Verification items for the finished model (mm, model axes). A direction names the side the tool comes from. Coordinates: 2 decimals unless noted, no trailing zeros. Write each loop counter-clockwise with the first axis right and the second up, starting at its lowest first coordinate (ties: lowest second). Pieces come first, ordered by that corner, then holes.
```python
from build123d import *

# Parameters (mm, degrees)
BASPROSKE_W          = 6
BASPROSKE_H          = 22
TOOTHCUT_DEPTH       = 32.685959036
TEETHCUTS_COUNT      = 20
TEETHCUTS_ANGLE      = 342
HUBNEAONESKE_R       = 11
HUBNEARONE_DEPTH     = 6.2500508
BORSKE_R             = 4
BORE_DEPTH           = 12.2500508
M2_CLEARANCE_HOLE1_D = 2.2


with BuildPart() as part:
    # BasProSke → Base-Revolve (revolve)
    with BuildSketch(Plane(origin=(0, 0, 0), x_dir=(1, 0, 0), z_dir=(0, 1, 0)), mode=Mode.PRIVATE) as base_revolve_sk:
        with Locations((3, 11)):
            Rectangle(BASPROSKE_W, BASPROSKE_H)
    revolve(base_revolve_sk.sketch.rotate(Axis((-10, 0, 0), (1, 0, 0)), 180), axis=Axis((-10, 0, 0), (1, 0, 0)))

    # TooCutSke → ToothCut (cut, through all)
    with BuildSketch(Plane(origin=(0, 0, 0), x_dir=(0, 0, -1), z_dir=(1, 0, 0))):
        with BuildLine():
            ThreePointArc((0.986171591, 17.471189616), (0, 17.499), (-0.986171591, 17.471189616))
            ThreePointArc((-0.986171591, 17.471189616), (-1.626916196, 19.798789858), (-2.932850173, 21.829260982))
            ThreePointArc((-2.932850173, 21.829260982), (0, 22.0254), (2.932850173, 21.829260982))
            ThreePointArc((2.932850173, 21.829260982), (1.626916196, 19.798789858), (0.986171591, 17.471189616))
        make_face()
    toothcut = extrude(amount=TOOTHCUT_DEPTH, mode=Mode.SUBTRACT)

    # TeethCuts: ToothCut ×20 about axis
    teethcuts_axis = Axis((-10, 0, 0), (1, 0, 0))
    for i in range(1, TEETHCUTS_COUNT):
        add(toothcut.rotate(teethcuts_axis, i * TEETHCUTS_ANGLE / (TEETHCUTS_COUNT - 1)), mode=Mode.SUBTRACT)

    # HubNeaOneSke → HubNearOne (add)
    with BuildSketch(Plane.ZY):
        with Locations(Location((0, 0, 0), (0, 0, 180))):
            Circle(HUBNEAONESKE_R)
    extrude(amount=HUBNEARONE_DEPTH)

    # BorSke → Bore (cut, symmetric)
    with BuildSketch(Plane(origin=(0, 0, 0), x_dir=(0, 0, -1), z_dir=(1, 0, 0))):
        with Locations(Location((0, 0, 0), (0, 0, 180))):
            Circle(BORSKE_R)
    extrude(amount=BORE_DEPTH, both=True, mode=Mode.SUBTRACT)

    # M2 Clearance Hole1 (through all)
    with Locations(Plane(origin=(6, 0, 0), x_dir=(0, 0, -1), z_dir=(1, 0, 0))):
        with Locations((0, 8), (5.656854249, 5.656854249), (8, 0), (5.656854249, -5.656854249), (0, -8), (-5.656854249, -5.656854249), (-8, 0), (-5.656854249, 5.656854249)):
            Hole(M2_CLEARANCE_HOLE1_D / 2)


solid = part.part
```
1. Sectioned sample at C-C, the plane z = -8. Record the boundary of the cut face in (x, y).
2. Material ranges on L1, parallel to Y at x = -2.75, z = 0; L2, parallel to Z at x = -1.25, y = 5; L3, parallel to Y at x = -5, z = 1, recorded low to high.
3. Gauge pin test, flat ends, axial feed: P1, Ø6, axis at y = -5.5, z = 17, coming from the -X side; P2, Ø5, axis at x = 0, y = 10, coming from the +Z side; P3, Ø4, axis at x = -4, y = 7, coming from the -Z side. Record the tip position at first contact, or that the pin passes through.
4. Sectioned sample at D-D, the plane x = -2.75. Give the number of separate pieces and of enclosed holes in the cut face, and give its area (3 significant figures).
5. Sectioned sample at A-A, the plane y = 0. Record the boundary of the cut face in (x, z).
6. Draft check along Y on faces 1 (the flat face through (6, 5, 0)), 2 (the cylindrical face through (-0.211, 6.747, -5.8)), 3 (the cylindrical face through (2.96, 7.63, -18.29)), 4 (the cylindrical face through (3.04, -9.99, -19.6)). Enter one of: pulls with the +Y half, pulls with the -Y half, needs draft (parallel to the pull), parting line crosses it, or undercut.
7. Tool access check on faces 5 (the cylindrical face through (2.96, -4.57, 19.35)), 6 (the cylindrical face through (2.96, 18.29, 7.63)), 7 (the cylindrical face through (2.958, -7.678, -18.341)). Record the directions out of +Z, -Z, +X, -X, +Y, -Y that give a thin tool (end or side, any length) a straight path to the whole face; none if there is none.
Outcome:
1. outline: (-6.25, -7.55) - (0, -7.55) - (0, -18.68) - (6, -18.68) - (6, -1.1) - (-6.25, -1.1) - close; (-6.25, 1.1) - (6, 1.1) - (6, 18.68) - (0, 18.68) - (0, 7.55) - (-6.25, 7.55) - close
2. L1: y = -11 to -9.1, -6.9 to -4, 4 to 6.9, 9.1 to 11
2. L2: z = -9.8 to -6.54, -4.77 to 4.77, 6.54 to 9.8
2. L3: y = -10.95 to -8.46, -7.54 to -3.87, 3.87 to 7.54, 8.46 to 10.95
3. P1: stops at x = 0
3. P2: stops at z = 19.84
3. P3: stops at z = -9.8
4. separate pieces: 1
4. enclosed holes: 9
4. area: 299 mm2
5. outline: (-6.25, -11) - (0, -11) - (0, -17.5) - (6, -17.5) - (6, -9.1) - (-6.25, -9.1) - close; (-6.25, -6.9) - (6, -6.9) - (6, -4) - (-6.25, -4) - close; (-6.25, 4) - (6, 4) - (6, 6.9) - (-6.25, 6.9) - close; (-6.25, 9.1) - (6, 9.1) - (6, 17.5) - (0, 17.5) - (0, 11) - (-6.25, 11) - close
6. face 1: needs draft
6. face 2: undercut
6. face 3: undercut
6. face 4: pulls with the -Y half
7. face 5: +X, -X
7. face 6: +X, -X, +Y
7. face 7: -Z, +X, -X
